Input: part model. Units: mm. Frame: model coordinates. Round coordinates to 2 decimals unless told otherwise and drop trailing zeros. Write each loop counter-clockwise with the first axis right and the second up, starting at its lowest first coordinate (ties: lowest second). Pieces come first, ordered by that corner, then holes. Notation, with made-up numbers: (53, -38.75) -> (91, -38.75) arc R17 ccw to (91, -30.75) -> close; hole circle Ø10 at (-31.5, 69.25). An arc over 180 degrees is marked (long way). Use CSV: the item, a comma, the result in double quotes.
```python
from build123d import *

# Parameters (mm, degrees)
F0_R     = 14.2875
F1_DEPTH = 6.35
F2_R     = 2.54
F3_DEPTH = 6.351


with BuildPart() as f1:
    # F0 (on Front) → F1 (new body)
    with BuildSketch(Plane.XZ):
        with BuildLine():
            Line((0, 38.1), (0, 0))
            Line((0, 0), (152.4, 0))
            Line((152.4, 0), (152.4, 38.1))
            ThreePointArc((152.4, 38.1), (149.718451, 49.459225), (142.24, 58.42))
            Line((142.24, 58.42), (91.44, 96.52))
            ThreePointArc((91.44, 96.52), (76.2, 101.6), (60.96, 96.52))
            Line((60.96, 96.52), (10.16, 58.42))
            ThreePointArc((10.16, 58.42), (2.681549, 49.459225), (0, 38.1))
        make_face()
        with Locations((76.2, 76.2)):
            Circle(F0_R, mode=Mode.SUBTRACT)
    extrude(amount=F1_DEPTH)

    # F2 (on face) → F3 (cut, through all)
    with BuildSketch(Plane.XZ.offset(6.35)):
        with Locations((12.927955, 38.1)):
            Circle(F2_R)
        with Locations((56.922045, 12.7)):
            Circle(F2_R)
        with Locations((95.477955, 12.7)):
            Circle(F2_R)
        with Locations((139.472045, 38.1)):
            Circle(F2_R)
    extrude(amount=-F3_DEPTH, mode=Mode.SUBTRACT)


solid = f1.part
```
Item 1: Section query A-A on x = 76.2. Return the cut outline in (y, z), plus the area to 3 significant figures.
Worked answers:
outline,"(-6.35, 0) -> (0, 0) -> (0, 61.91) -> (-6.35, 61.91) -> close; (-6.35, 90.49) -> (0, 90.49) -> (0, 101.6) -> (-6.35, 101.6) -> close"
area,"464 mm²"
Item 2: Line query: line 1 (Z direction, x = 76, y = -0.5); line 2 (Z direction, x = 87.5, y = -3.5); line 3 (Z direction, x = 7, y = -4.5). Output: solid intervals per line, ascending.
Worked answers:
line 1,"z = 0 to 61.91, 90.49 to 101.6"
line 2,"z = 0 to 67.46, 84.94 to 98.95"
line 3,"z = 0 to 55.61"
Item 3: Section query C-C on y = -1.75. Return the cut outline in (x, z) (1 decimal), plus the area to 3 significant figures.
Worked answers:
outline,"(0, 0) -> (152.4, 0) -> (152.4, 38.1) arc R25.4 ccw to (142.2, 58.4) -> (91.4, 96.5) arc R25.4 ccw to (61, 96.5) -> (10.2, 58.4) arc R25.4 ccw to (0, 38.1) -> close; hole circle Ø5.1 at (12.9, 38.1); hole circle Ø5.1 at (56.9, 12.7); hole circle Ø28.6 at (76.2, 76.2); hole circle Ø5.1 at (95.5, 12.7); hole circle Ø5.1 at (139.5, 38.1)"
area,"11,300 mm²"
Item 4: First-contact query: pin 1 Ø2 at (y, z) = (-1.5, 86.5) entering from -X. Flat tip, straight axial feed; report the tip coordinate or a pass-through.
Worked answers:
pin 1,"stops at x = 46.27"
Item 5: Pull-direction query (X, two-part tool) for faces 1 (the face through (74.34, -3.131, 90.366)), 2 (the face through (141.895, -3.219, 38.863)), 3 (the face through (117.2, -3.1, 77.2)), 4 (the face through (2.756, -3.131, 49.606)); classes: +X half, -X half, draft (parallel to the pull), parting line (faces both ways), or undercut.
Worked answers:
face 1,"undercut"
face 2,"undercut"
face 3,"+X half"
face 4,"-X half"
Item 6: Section query D-D on z = 79. Return the cut outline in (x, y), plus the area to 3 significant figures.
Worked answers:
outline,"(37.6, -6.35) -> (62.19, -6.35) -> (62.19, 0) -> (37.6, 0) -> close; (90.21, -6.35) -> (114.8, -6.35) -> (114.8, 0) -> (90.21, 0) -> close"
area,"312 mm²"
Item 7: Section query B-B on z = 12.7. Return the cut outline in (x, y), plus the area to 3 significant figures.
Worked answers:
outline,"(0, -6.35) -> (54.38, -6.35) -> (54.38, 0) -> (0, 0) -> close; (59.46, -6.35) -> (92.94, -6.35) -> (92.94, 0) -> (59.46, 0) -> close; (98.02, -6.35) -> (152.4, -6.35) -> (152.4, 0) -> (98.02, 0) -> close"
area,"903 mm²"
